```python
from build123d import *

# Parameters (mm, degrees)
SKETCH_1_W          = 20
SKETCH_1_H          = 20
SKETCH_1_W_2        = 17
SKETCH_1_H_2        = 17
EXTRUDE_1_DEPTH     = 616
SKETCH_4_R          = 2.5
CUT_EXTRUDE_3_DEPTH = 20
SKETCH_5_R          = 2
CUT_EXTRUDE_4_DEPTH = 20


with BuildPart() as part:
    # 草图1 → 凸台-拉伸1 (new body)
    with BuildSketch(Plane.XY):
        Rectangle(SKETCH_1_W, SKETCH_1_H)
        Rectangle(SKETCH_1_W_2, SKETCH_1_H_2, mode=Mode.SUBTRACT)
    extrude(amount=EXTRUDE_1_DEPTH)

    # 草图4 → 切除-拉伸3 (cut)
    with BuildSketch(Plane.XZ.offset(10)):
        with Locations(Location((4, 13, 0), (0, 0, 270))):
            Circle(SKETCH_4_R)
        with Locations(Location((4, 43, 0), (0, 0, 270))):
            Circle(SKETCH_4_R)
        with Locations(Location((4, 603, 0), (0, 0, 270))):
            Circle(SKETCH_4_R)
        with Locations(Location((4, 573, 0), (0, 0, 270))):
            Circle(SKETCH_4_R)
    extrude(amount=-CUT_EXTRUDE_3_DEPTH, mode=Mode.SUBTRACT)

    # 草图5 → 切除-拉伸4 (cut)
    with BuildSketch(Plane.XZ.offset(10)):
        with Locations(Location((0, 230, 0), (0, 0, 270))):
            Circle(SKETCH_5_R)
        with Locations(Location((0, 386, 0), (0, 0, 270))):
            Circle(SKETCH_5_R)
    extrude(amount=-CUT_EXTRUDE_4_DEPTH, mode=Mode.SUBTRACT)


solid = part.part
```
Check sheet for the modelled part. Datum: model origin and axes. Units: mm. A direction names the side the tool comes from. Round coordinates to 2 decimals unless told otherwise and drop trailing zeros. Loops run counter-clockwise (first coordinate to the right, second up) from the corner with the lowest first, then second, coordinate; pieces in that order, holes last. Notation, with made-up numbers: (-15.5, 60) - (4.5, 60) arc R21 cw to (4.5, 72) - close; hole circle Ø8 at (36, 33.25). An arc over 180 degrees is marked (long way). Answer as a JSON object with one key per item and string values. Group by question number.
Q1. Sectioned sample at A-A, the plane y = 4.25. Enter the section's corners in (x, z).
Q2. Scan lines: line 1 along X through (y, z) = (-7, 407.5); line 2 along X through (y, z) = (9.3, 573). Record each from-to range of solid material in increasing order. Write a range as [from, to].
Q3. Gauge pin test, flat end, axial feed: P1, Ø10, axis at x = 1.5, y = 1.5, coming from the -Z side. Record the tip position at first contact, or that the pin passes through.
Q4. Sectioned sample at B-B, the plane z = 546. Enter the section's corners in (x, y).
Q5. Mould release check, pull along X, two halves, no side actions. Record for faces 3 (the face through (0, -8.5, 304)), 4 (the face through (-10, 0, 304)), 5 (the face through (-9, 0, 0)): released by +X, released by -X, zero draft, split by the parting line, or undercut.
Q6. Set-up check for faces 1 (the face through (0, 8.5, 304)), 2 (the face through (0, 10, 304)): record each of +Z, -Z, +X, -X, +Y, -Y from which the full face is reachable in a straight line by a thin tool's end or side.
Solution:
{
 "1": {"outline": "(-10, 0) - (-8.5, 0) - (-8.5, 616) - (-10, 616) - close; (8.5, 0) - (10, 0) - (10, 616) - (8.5, 616) - close"},
 "2": {"line 1": "x = [-10, -8.5], [8.5, 10]", "line 2": "x = [-10, 1.5], [6.5, 10]"},
 "3": {"P1": "passes through"},
 "4": {"outline": "(-10, -10) - (10, -10) - (10, 10) - (-10, 10) - close; hole (-8.5, -8.5) - (8.5, -8.5) - (8.5, 8.5) - (-8.5, 8.5) - close"},
 "5": {"face 3": "undercut", "face 4": "released by -X", "face 5": "zero draft"},
 "6": {"face 1": "+Z, -Z", "face 2": "+Z, -Z, +X, -X, +Y"}
}
